Model file for the job. Use its own axes, mm. Face numbers are marked on the shaded views. A direction names the side the tool comes from. Round coordinates to 2 decimals unless told otherwise and drop trailing zeros. Write each loop counter-clockwise with the first axis right and the second up, starting at its lowest first coordinate (ties: lowest second). Pieces come first, ordered by that corner, then holes. Notation, with made-up numbers: (-0.5, -12) - (57.5, -12) arc R19 ccw to (57.5, 18) - close; hole circle Ø9 at (9.25, -16). An arc over 180 degrees is marked (long way). Answer as a JSON object with one key per item and string values. Group by question number.
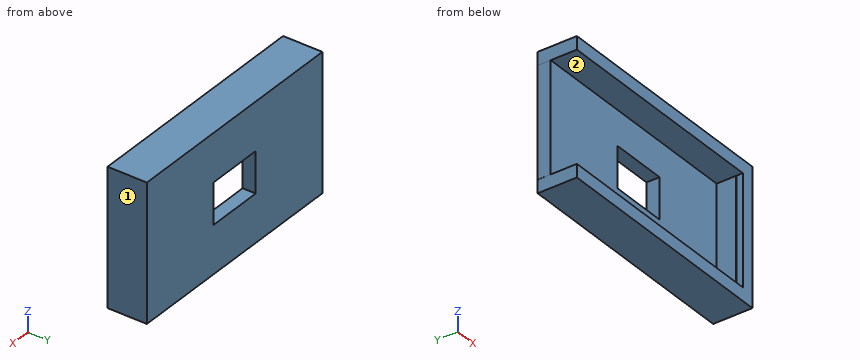
Autodesk Fusion 360 part; units mm, degrees
sketch "Sketch1" plane through (0, 0, 0) normal (0, 1, 0) x (1, 0, 0)
  line L0 (0, 0) -> (25.9, 0)
  line L1 (25.9, 0) -> (25.9, 13.45)
  line L2 (25.9, 13.45) -> (0, 13.45)
  line L3 (0, 13.45) -> (0, 0)
  line L4 (-1.6, 15.05) -> (27.5, 15.05)
  line L5 (27.5, 15.05) -> (27.5, -1.6)
  line L6 (27.5, -1.6) -> (-1.6, -1.6)
  line L7 (-1.6, -1.6) -> (-1.6, 15.05)
  dimension "d1" = 25.9
  dimension "d2" = 13.45
  dimension "d3" = 1.6
  dimension "d4" = 1.6
  dimension "d5" = 1.6
  dimension "d6" = 1.6
extrude "Extrude1" add sketch "Sketch1" along normal blind 1.6 contours L0 L1 L2 L3 | L4 L5 L6 L7
extrude "Extrude2" add sketch "Sketch1" along normal blind 4.8
extrude "Extrude3" cut 1 faces at (0, 2.6667, -8.9667) along direction (-1, 0, 0) blind 1.6002
sketch "Sketch2" plane through (25.9, 0, 0) normal (-1, 0, 0) x (0, 0, 1)
  line L0 (-13.45, 1.6) -> (0, 1.6)
  line L1 (0, 1.6) -> (0, 4.8)
  line L2 (0, 4.8) -> (-13.45, 4.8)
  line L3 (-13.45, 4.8) -> (-13.45, 1.6)
  line L4 (-13.45, 4.8) -> (0, 4.8)
  line L5 (0, 4.8) -> (0, 3.2)
  line L6 (0, 3.2) -> (-13.45, 3.2)
  line L7 (-13.45, 3.2) -> (-13.45, 4.8)
  dimension "d13" = 1.6
extrude "Extrude4" add sketch "Sketch2" along normal blind 27.5082 contours L1 L2 L3 L4 L5 L6 L7
sketch "Sketch3" plane through (0, 4.8, 0) normal (0, 1, 0) x (-1, 0, 0)
  line L0 (1.6, 0) -> (1.6, 1.6)
  line L1 (1.6, 1.6) -> (-27.5, 1.6)
  line L2 (-27.5, 1.6) -> (-27.5, -15.05)
  line L3 (-27.5, -15.05) -> (1.6, -15.05)
  line L4 (1.6, -15.05) -> (1.6, -13.45)
  line L5 (1.6, -13.45) -> (1.6082, -13.45)
  line L6 (1.6082, -13.45) -> (1.6082, 0)
  line L7 (1.6082, 0) -> (1.6, 0)
  line L8 (-9.4458, -9.2312) -> (-16.4458, -9.2312)
  line L9 (-16.4458, -9.2312) -> (-16.4458, -4.2312)
  line L10 (-16.4458, -4.2312) -> (-9.4458, -4.2312)
  line L11 (-9.4458, -4.2312) -> (-9.4458, -9.2312)
  line L12 (-9.4458, -9.2312) -> (-12.9458, -9.2312)
  line L13 (-12.9458, -9.2312) -> (-12.9458, -6.7312)
  line L14 (-12.9458, -6.7312) -> (-9.4458, -6.7312)
  line L15 (-9.4458, -6.7312) -> (-9.4458, -9.2312)
  dimension "d16" = 7
  dimension "d17" = 5
  dimension "d18" = 16.65
  dimension "d19" = 29.1
  dimension "d20" = 14.5542
  dimension "d21" = 8.3312
extrude "Extrude5" cut sketch "Sketch3" against normal blind 2.54 contours L8 L11 L12 L13 L14 L15 | L8 L9 L10 L11 L13 L14
extrude "Extrude6" cut 1 faces at (16.7333, 1.6, -4.4833) along direction (0, -1, 0) blind 0.8
sketch "Sketch4" plane through (-1.6, 0, 0) normal (-1, 0, 0) x (0, 0, 1)
  line L0 (0, 3.2) -> (0, 0.8)
  line L1 (0, 0.8) -> (-13.45, 0.8)
  line L2 (-13.45, 0.8) -> (-13.45, 3.2)
  line L3 (-13.45, 3.2) -> (-13.45, 4.8)
  line L4 (-13.45, 4.8) -> (-15.05, 4.8)
  line L5 (-15.05, 4.8) -> (-15.05, 0)
  line L6 (-15.05, 0) -> (1.6, 0)
  line L7 (1.6, 0) -> (1.6, 4.8)
  line L8 (1.6, 4.8) -> (0, 4.8)
  line L9 (0, 4.8) -> (0, 3.2)
  line L10 (-13.45, 0.8) -> (0, 0.8)
  line L11 (0, 0.8) -> (0, 0)
  line L12 (0, 0) -> (-13.45, 0)
  line L13 (-13.45, 0) -> (-13.45, 0.8)
extrude "Extrude7" cut sketch "Sketch4" against normal blind 27.5082 contours L1 L6 L10 L11 L12 L13
equation "d9 = 1.6 * 3 mm"
equation "d20 = ( 1.146 / 2 ) * 1 in"
equation "d21 = ( 0.656 / 2 ) * 1 in"
equation "d24 = -( 1.6 / 2 ) * 1 mm"
(1) Flat gauge pins, fed straight in: pin 1 (1.8 mm diameter, centred on y = 2, z = -14.5, fed in from -X); pin 2 (0.7 mm diameter, centred on y = 2.5, z = -7.5, fed in from -X); pin 3 (8 mm diameter, centred on x = 4.5, z = -9, fed in from -Y). Where does each tip first touch, or does it go through?
(2) Slice it at B-B (x = 10.75). Write the cut outline in (y, z).
(3) Slice it at D-D (x = 25). Write the cut outline in (y, z), then the cut area to 3 significant figures.
(4) Drill centre lines: line 1 (X direction, y = 3.8, z = -4.5); line 2 (Z direction, x = 7, y = 2); line 3 (X direction, y = 0.7, z = -9). Where is each one in solid material? Low to high. Write a range as from..to.
(5) 3-axis set-ups, long thin cutter, end or side, ignore diameter. For the marked faces 1 and 2: which of +Z, -Z, +X, -X, +Y, -Y reach the whole face in a straight line?
Answer:
{
 "1": {"pin 1": "x = -1.6", "pin 2": "x = 25.9", "pin 3": "y = 3.2"},
 "2": {"outline": "(0, -15.05) - (4.8, -15.05) - (4.8, -9.23) - (3.2, -9.23) - (3.2, -13.45) - (0, -13.45) - close; (0, 0) - (3.2, 0) - (3.2, -4.23) - (4.8, -4.23) - (4.8, 1.6) - (0, 1.6) - close"},
 "3": {"outline": "(0, -15.05) - (4.8, -15.05) - (4.8, 1.6) - (0, 1.6) - (0, 0) - (3.2, 0) - (3.2, -13.45) - (0, -13.45) - close", "area": "36.9 mm²"},
 "4": {"line 1": "-1.61..9.45, 16.45..27.5", "line 2": "-15.05..-13.45, 0..1.6", "line 3": "25.91..27.5"},
 "5": {"face 1": "+Z, -Z, +X, +Y, -Y", "face 2": "-X, -Y"}
}
